The listing builds one solid part. Answer for the finished solid, in the listing's coordinates (mm). A direction names the side the tool comes from. Give positions to 0.01 mm unless a question says otherwise; leave off trailing zeros. Write each loop counter-clockwise with the first axis right and the second up, starting at its lowest first coordinate (ties: lowest second). Pieces come first, ordered by that corner, then holes. Notation, with made-up numbers: (-14.5, 86.5) -> (26.5, 86.5) arc R32 ccw to (26.5, 112.5) -> close; hole circle Ø2 at (81.5, 68). An arc over 180 degrees is marked (long way). Put each result on its own line as item: value. Start each with the question number.
1) A cutting plane is placed at D-D (x = -8). Write down the section's boundary in (y, z), then the cut area to 3 significant figures.
2) Flat-ended cylindrical pins translate along their axes: pin 1 Ø5 at (x, z) = (-13, 13) entering from +Y; pin 2 Ø4 at (x, y) = (-13, -1.5) entering from +Z; pin 3 Ø3.5 at (x, y) = (-37, 0) entering from +Z. Find the tip coordinate at first contact, or state that the pin passes through.
3) A cutting plane is placed at C-C (x = -22.5). Write down the section's boundary in (y, z), then the cut area to 3 significant figures.
4) Find the intervals of material crossed by line 1 along Y through (x, z) = (-37, 3.75); line 2 along X through (y, z) = (0, 5.25); line 3 along X through (y, z) = (0, 4), in increasing order. Write a range as from..to.
5) For faces 1 (the flat face through (-6, 0, 10)), 2 (the flat face through (-6, 0, 0)), 3 (the cylindrical face through (-6.85, 6.05, 9.57)), 4 (the cylindrical face through (-22.324, -0.035, 7.998)), determine the directions among +Z, -Z, +X, -X, +Y, -Y from which every point of the face is accessible in a straight line to the end or side of a thin tool.
6) For a pull along X with two mould halves and no side action, classify faces 5 (the cylindrical face through (-44.57, -6.05, 4.31)), 6 (the cylindrical face through (-22.65, -4.47, 7)), 7 (the flat face through (-40, 0, 10)) as released by +X, released by -X, zero draft, split by the parting line, or undercut.
7) A cutting plane is placed at B-B (y = 0). Write down the section's boundary in (x, z), then the cut area to 3 significant figures.
8) A cutting plane is placed at A-A (z = 3). Write down the section's boundary in (x, y).
Solid Edge part; units mm, degrees
sketch "Sketch1" plane through (0, 0, 0) normal (1, 0, 0) x (0, 1, 0)
  line L0 (6.5, 10) -> (6.5, 0)
  line L1 (6.5, 0) -> (-6.5, 0)
  line L2 (-6.5, 0) -> (-6.5, 10)
  line L3 (-6.5, 10) -> (6.5, 10)
extrude "Protrusion1" add sketch "Sketch1" against normal blind 45
fillet "Redondeo_1" radius 1.5 4 edges at (0, -6.5, 5) (-45, -6.5, 5) (-45, 6.5, 5) (0, 6.5, 5)
sketch "Sketch2" plane through (-22.25, 6.5, 6.5) normal (0, 1, 0) x (0, 0, -1)
  circle A0 centre (6.5, 0.25) radius 7
extrude "Cutout1" cut sketch "Sketch2" against normal through all
sketch "Sketch3" plane through (-22.25, 6.5, 6.5) normal (0, 1, 0) x (-1, 0, 0)
  line L0 (-5.4308, 8) -> (5.9308, 8)
  line L1 (5.9308, 8) -> (11.25, 3.5)
  line L2 (11.25, 3.5) -> (-10.75, 3.5)
  line L3 (-10.75, 3.5) -> (-5.4308, 8)
extrude "ProtrusiónExtruida_2" add sketch "Sketch3" against normal blind 13
fillet "Redondeo_2" radius 1.5 17 edges at (-6.5, 6.5, 10) (-0.4393, 6.0607, 10) (0, 0, 10) (-0.4393, -6.0607, 10) (-6.5, -6.5, 10) (-38.5, 6.5, 10) (-45, 0, 10) (-44.5607, -6.0607, 10) (-38.5, -6.5, 10) (-14.1596, 6.5, 12.25) (-14.1596, -6.5, 12.25) (-16.8192, 0, 14.5) (-22.5, 6.5, 14.5) (-28.1808, 0, 14.5) (-22.5, -6.5, 14.5) (-30.8404, -6.5, 12.25) (-30.8404, 6.5, 12.25)
sketch "Sketch4" plane through (-7.25, 0, 10) normal (0, 0, 1) x (0, 1, 0)
  circle A0 centre (0, 0.75) radius 1.5
  circle A1 centre (0, 29.75) radius 1.5
extrude "Cutout2" cut sketch "Sketch4" against normal through all
sketch "Sketch5" plane through (0, 0, 0) normal (0, 0, 1) x (1, 0, 0)
  line L0 (-22.5, 2.5) -> (-14.5, 2.5)
  line L1 (-14.5, 2.5) -> (-14.5, -2.5)
  line L2 (-14.5, -2.5) -> (-22.5, -2.5)
  line L3 (-22.5, -2.5) -> (-22.5, 2.5)
revolve "RevolvedCutout1" cut sketch "Sketch5" angle 360 about axis through (-22.5, 8, 0) along (0, -1, 0)
Reply:
1. outline: (-6.5, 0) -> (-1.5, 0) -> (-1.5, 10) -> (-5, 10) arc R1.5 ccw to (-6.5, 8.5) -> close; (1.5, 0) -> (6.5, 0) -> (6.5, 8.5) arc R1.5 ccw to (5, 10) -> (1.5, 10) -> close
1. area: 99.0 mm2
2. pin 1: stops at y = 6.47
2. pin 2: stops at z = 12.96
2. pin 3: stops at z = 10
3. outline: (-6.5, 7) -> (-2.5, 7) -> (-2.5, 8) -> (2.5, 8) -> (2.5, 7) -> (6.5, 7) -> (6.5, 13) arc R1.5 ccw to (5, 14.5) -> (-5, 14.5) arc R1.5 ccw to (-6.5, 13) -> close
3. area: 91.5 mm2
4. line 1: y = -6.5..-1.5, 1.5..6.5
4. line 2: x = -45..-38.5, -35.5..-28.54, -16.46..-9.5, -6.5..0
4. line 3: x = -45..-38.5, -35.5..-29.43, -15.57..-9.5, -6.5..0
5. face 1: +Z, +X, +Y, -Y
5. face 2: -Z, +X, -X, +Y, -Y
5. face 3: +Z, +X, +Y
5. face 4: -Z
6. face 5: released by -X
6. face 6: undercut
6. face 7: zero draft
7. outline: (-45, 0) -> (-38.5, 0) -> (-38.5, 10) -> (-43.5, 10) arc R1.5 ccw to (-45, 8.5) -> close; (-35.5, 0) -> (-30.5, 0) arc R8 cw to (-14.5, 0) -> (-9.5, 0) -> (-9.5, 10) -> (-11.5, 10) -> (-16.4, 14.15) arc R1.5 ccw to (-17.37, 14.5) -> (-27.63, 14.5) arc R1.5 ccw to (-28.6, 14.15) -> (-33.5, 10) -> (-35.5, 10) -> close; (-6.5, 0) -> (0, 0) -> (0, 8.5) arc R1.5 ccw to (-1.5, 10) -> (-6.5, 10) -> close
7. area: 363 mm2
8. outline: (-45, -5) arc R1.5 ccw to (-43.5, -6.5) -> (-28.82, -6.5) -> (-28.82, -2.5) -> (-29.92, -2.5) -> (-29.92, 2.5) -> (-28.82, 2.5) -> (-28.82, 6.5) -> (-43.5, 6.5) arc R1.5 ccw to (-45, 5) -> close; (-16.18, -6.5) -> (-1.5, -6.5) arc R1.5 ccw to (0, -5) -> (0, 5) arc R1.5 ccw to (-1.5, 6.5) -> (-16.18, 6.5) -> (-16.18, 2.5) -> (-15.08, 2.5) -> (-15.08, -2.5) -> (-16.18, -2.5) -> close; hole circle Ø3 at (-37, 0); hole circle Ø3 at (-8, 0)
